Part print with two shaded views. Sizes in mm from the minimum x, y, z corner. A direction names the side the tool comes from. Round coordinates to 2 decimals unless told otherwise and drop trailing zeros. Write each loop counter-clockwise with the first axis right and the second up, starting at its lowest first coordinate (ties: lowest second). Pieces come first, ordered by that corner, then holes. Notation, with made-up numbers: (-6, 36.5) -> (37, 36.5) arc R8 cw to (37, 46.5) -> close; hole circle Ø4 at (-10, 47). An arc over 180 degrees is marked (long way). Return JSON: item names as keys, results as strings. Group by question number.
(1) Tool access for the marked faces 1, 2 and 3: list every direction of +Z, -Z, +X, -X, +Y, -Y with a clear straight run to the whole face (end or side of a thin tool).
(2) Drill centre lines: L1, parallel to Z at x = 6, y = 11.5; L2, parallel to Y at x = 6, z = 22; L3, parallel to Z at x = 21, y = 11. Where is each one in solid material? Low to high. Write a range as from..to.
(3) Saw through at D-D (y = 21). List the corners of the cut face in (x, z), plus the area to 3 significant figures.
(4) Saw through at B-B (x = 29). List the corners of the cut face in (y, z), plus the area to 3 significant figures.
(5) Drop flat-ended pins along their axis: pin 1 Ø9.5 at (x, z) = (44, 18.5) entering from -Y; pin 2 Ø3 at (y, z) = (4, 21) entering from -X (3 decimals); pin 3 Ø9.5 at (y, z) = (6.5, 17.5) entering from +X; pin 4 Ø5 at (y, z) = (18.5, 24) entering from +X. Give the stop position or say it passes through.
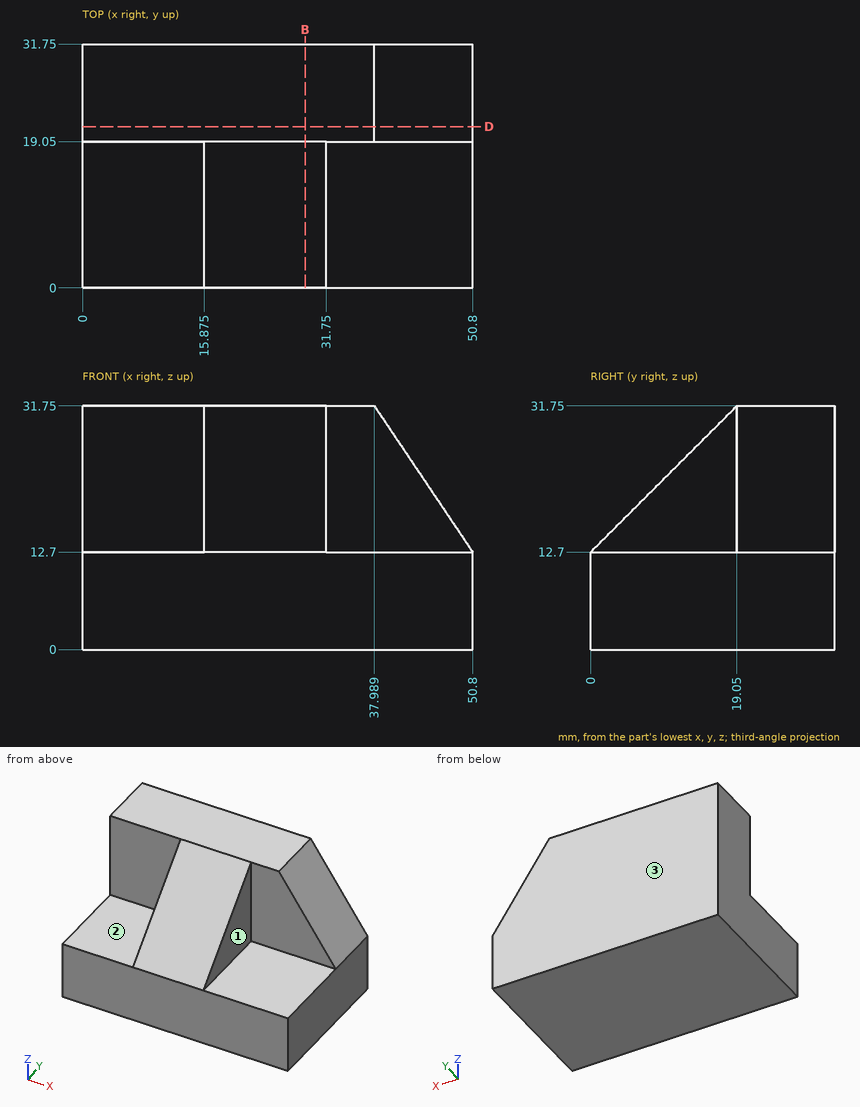
Computed values:
{
 "1": {"face 1": "+Z, +X, -Y", "face 2": "+Z, -X, -Y", "face 3": "+Z, -Z, +X, -X, +Y"},
 "2": {"L1": "0..12.7", "L2": "19.05..31.75", "L3": "0..23.7"},
 "3": {"outline": "(0, 0) -> (50.8, 0) -> (50.8, 12.7) -> (37.99, 31.75) -> (0, 31.75) -> close", "area": "1,490 mm2"},
 "4": {"outline": "(0, 0) -> (31.75, 0) -> (31.75, 31.75) -> (19.05, 31.75) -> (0, 12.7) -> close", "area": "827 mm2"},
 "5": {"pin 1": "y = 19.05", "pin 2": "through", "pin 3": "x = 31.75", "pin 4": "x = 44.84"}
}
